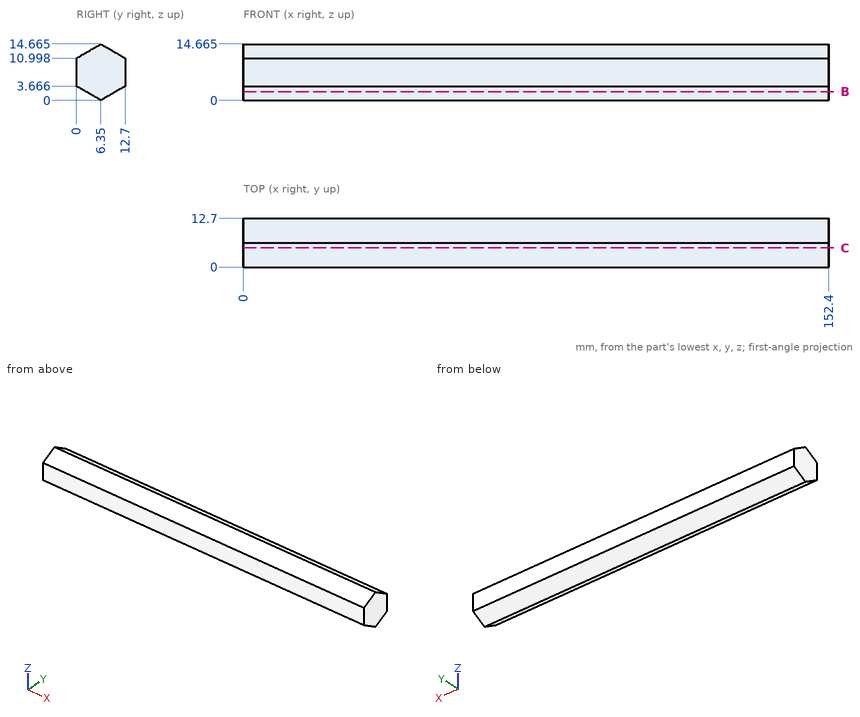
Study the drawing (mm; zero at the part's minimum x, y, z) and answer. Coordinates: 2 decimals unless noted, no trailing zeros. Write each loop counter-clockwise with the first axis right and the second up, starting at its lowest first coordinate (ties: lowest second). Pieces come first, ordered by that corner, then holes.
Q1. Find the intervals of material crossed by line 1 (Y direction, x = 110.5, z = 11.25) (1 decimal); line 2 (Z direction, x = 131, y = 8.5) (1 decimal); line 3 (Z direction, x = 7.5, y = 11) (1 decimal), in increasing order.
Q2. Each of these flat-tipped pins is pushed along its axis until it touches: pin 1 Ø1 at (x, z) = (24, 12.5) entering from +Y (1 decimal); pin 2 Ø5 at (x, y) = (41.5, 3) entering from -Z; pin 3 Ø6 at (x, y) = (60.5, 9.5) entering from -Z. Where does it stop, or does it pass through?
Q3. A cutting plane is placed at B-B, the plane z = 2.25. Give the vertices of the cut face in (x, y), then the cut area to 3 significant figures.
Q4. A cutting plane is placed at C-C, the plane y = 5. Give the vertices of the cut face in (x, z) (1 decimal), then the cut area to 3 significant figures.
Findings below:
1. line 1: y = 0.4 to 12.3
1. line 2: z = 1.2 to 13.4
1. line 3: z = 2.7 to 12
2. pin 1: stops at y = 11
2. pin 2: stops at z = 0.49
2. pin 3: stops at z = 0.09
3. outline: (0, 2.45) - (152.4, 2.45) - (152.4, 10.25) - (0, 10.25) - close
3. area: 1,190 mm2
4. outline: (0, 0.8) - (152.4, 0.8) - (152.4, 13.9) - (0, 13.9) - close
4. area: 2,000 mm2
